Verification items for the finished model (mm, model axes). A direction names the side the tool comes from. Give positions to 0.01 mm unless a question says otherwise; leave off trailing zeros. Loops run counter-clockwise (first coordinate to the right, second up) from the corner with the lowest first, then second, coordinate; pieces in that order, holes last. Notation, with made-up numbers: (65.25, 65.5) - (94.25, 65.5) arc R16 cw to (94.25, 85.5) - close; hole circle Ø9 at (-34.75, -8.5). An arc over 180 degrees is marked (long way). One line per item, written item: value. Start each with the question number.
1. Sectioned sample at B-B (x = -93). Record the cut outline in (y, z), plus the area to 3 significant figures.
2. Mould release check, pull along Z, two halves, no side actions. Record for faces 1 (the flat face through (192, 6, 2)), 2 (the flat face through (-3, 8, 112)), 3 (the flat face through (-3, 9, 110)): pulls with the +Z half, pulls with the -Z half, needs draft (parallel to the pull), parting line crosses it, or undercut.
3. Gauge pin test, flat end, axial feed: pin 1 (6 mm diameter, centred on x = -90, z = -50, fed in from +Y). Record the tip position at first contact, or that the pin passes through.
4. Access from +Z, -Z, +X, -X, +Y, -Y to the whole of each face (thin tool, end or side, straight path). Record for faces 4 (the flat face through (-190, 11, 2)), 5 (the flat face through (-3, 0, -2)).
5. Sectioned sample at A-A (z = 80). Record the cut outline in (x, y), plus the area to 3 significant figures.
6. Scan lines: L1, parallel to X at y = 6.5, z = 101.5; L2, parallel to Z at x = 20.5, y = 16; L3, parallel to Y at x = 190.45, z = -95. Record each from-to range of solid material in increasing order. Write a range as [from, to].
from build123d import *

# Parameters (mm, degrees)
SKETCH_1_W          = 384
SKETCH_1_H          = 224
EXTRUDE_1_DEPTH     = 2
SKETCH_2_W          = 384
SKETCH_2_H          = 224
SKETCH_2_W_2        = 380
SKETCH_2_H_2        = 220
EXTRUDE_2_DEPTH     = 15
SKETCH_3_R          = 2.5
CUT_EXTRUDE_1_DEPTH = 296.514805044
SKETCH_4_R          = 2.5
CUT_EXTRUDE_2_DEPTH = 401.36108702


with BuildPart() as part:
    # 草图1 → 凸台-拉伸1 (new body)
    with BuildSketch(Plane(origin=(0, 0, 0), x_dir=(1, 0, 0), z_dir=(0, 1, 0))):
        Rectangle(SKETCH_1_W, SKETCH_1_H)
    extrude(amount=EXTRUDE_1_DEPTH)

    # 草图2 → 凸台-拉伸2 (add)
    with BuildSketch(Plane(origin=(0, 2, 0), x_dir=(1, 0, 0), z_dir=(0, 1, 0))):
        Rectangle(SKETCH_2_W, SKETCH_2_H)
        Rectangle(SKETCH_2_W_2, SKETCH_2_H_2, mode=Mode.SUBTRACT)
    extrude(amount=EXTRUDE_2_DEPTH)

    # 草图3 → 切除-拉伸1 (cut, through all)
    with BuildSketch(Plane(origin=(0, 0, -112), x_dir=(-1, 0, 0), z_dir=(0, 0, -1))):
        with Locations((-175, 8.5)):
            Circle(SKETCH_3_R)
        with Locations((-58.33, 8.5)):
            Circle(SKETCH_3_R)
        with Locations((58.34, 8.5)):
            Circle(SKETCH_3_R)
        with Locations((175.01, 8.5)):
            Circle(SKETCH_3_R)
    extrude(amount=-CUT_EXTRUDE_1_DEPTH, mode=Mode.SUBTRACT)

    # 草图4 → 切除-拉伸2 (cut, through all)
    with BuildSketch(Plane(origin=(192, 0, 0), x_dir=(0, 0, -1), z_dir=(1, 0, 0))):
        with Locations((-95, 8.5)):
            Circle(SKETCH_4_R)
        with Locations((0, 8.5)):
            Circle(SKETCH_4_R)
        with Locations((95, 8.5)):
            Circle(SKETCH_4_R)
    extrude(amount=-CUT_EXTRUDE_2_DEPTH, mode=Mode.SUBTRACT)


solid = part.part
Results are:
1. outline: (0, -112) - (17, -112) - (17, -110) - (2, -110) - (2, 110) - (17, 110) - (17, 112) - (0, 112) - close
1. area: 508 mm^2
2. face 1: needs draft
2. face 2: pulls with the +Z half
2. face 3: undercut
3. pin 1: stops at y = 2
4. face 4: +Y
4. face 5: +Z, -Z, +X, -X, -Y
5. outline: (-192, 0) - (192, 0) - (192, 17) - (190, 17) - (190, 2) - (-190, 2) - (-190, 17) - (-192, 17) - close
5. area: 828 mm^2
6. L1: x = [-192, -190], [190, 192]
6. L2: z = [-112, -110], [110, 112]
6. L3: y = [0, 6], [11, 17]
